```python
from build123d import *

# Parameters (mm, degrees)
F0_W     = 63.5
F0_H     = 508
F1_DEPTH = 19.05
F2_W     = 44.45
F2_H     = 508
F3_DEPTH = 19.05


with BuildPart() as f1:
    # F0 (on Front) → F1 (new body)
    with BuildSketch(Plane.XZ):
        Rectangle(F0_W, F0_H)
    extrude(amount=F1_DEPTH)

    # F2 (on face) → F3 (join)
    with BuildSketch(Plane.YZ.offset(31.75)):
        with Locations((-41.275, 0)):
            Rectangle(F2_W, F2_H)
    extrude(amount=-F3_DEPTH)


solid = f1.part
```
Read the model definition and answer for the solid it produces. Units are mm, in the model's axes. A direction names the side the tool comes from. Give positions to 0.01 mm unless a question says otherwise; leave off trailing zeros. Loops run counter-clockwise (first coordinate to the right, second up) from the corner with the lowest first, then second, coordinate; pieces in that order, holes last.
Item 1: For faces 1 (the flat face through (31.75, -32, 4)), 2 (the flat face through (-10, -19.05, 4)), determine the directions among +Z, -Z, +X, -X, +Y, -Y from which every point of the face is accessible in a straight line to the end or side of a thin tool.
Item 2: The part is cut by section B-B (y = -46.5). Write down the section's boundary in (x, z), and give its area (3 significant figures).
Item 3: The part is cut by section C-C (x = -14). Write down the section's boundary in (y, z), and give its area (3 significant figures).
Item 4: The part is cut by section A-A (z = -181). Write down the section's boundary in (x, y), and give its area (3 significant figures).
Item 5: Each of these flat-tipped pins is pushed along its axis until it touches: pin 1 Ø8 at (x, z) = (-11.5, 201) entering from -Y; pin 2 Ø2 at (x, z) = (19, 186) entering from +Y; pin 3 Ø3 at (x, z) = (-2.5, 82.5) entering from -Y. Where does it stop, or does it pass through?
Item 6: Find the intervals of material crossed by line 1 along Y through (x, z) = (-11.5, -55); line 2 along X through (y, z) = (-22.5, -76), in increasing order.
Taken from the geometry:
1. face 1: +Z, -Z, +X, +Y, -Y
1. face 2: +Z, -Z, -X, -Y
2. outline: (12.7, -254) - (31.75, -254) - (31.75, 254) - (12.7, 254) - close
2. area: 9,680 mm2
3. outline: (-19.05, -254) - (0, -254) - (0, 254) - (-19.05, 254) - close
3. area: 9,680 mm2
4. outline: (-31.75, -19.05) - (12.7, -19.05) - (12.7, -63.5) - (31.75, -63.5) - (31.75, 0) - (-31.75, 0) - close
4. area: 2,060 mm2
5. pin 1: stops at y = -19.05
5. pin 2: stops at y = 0
5. pin 3: stops at y = -19.05
6. line 1: y = -19.05 to 0
6. line 2: x = 12.7 to 31.75
